from build123d import *

# Parameters (mm, degrees)
SKETCH_1_W          = 37.5
SKETCH_1_H          = 37.5
EXTRUDE_1_DEPTH     = 82
SKETCH_2_W          = 57
SKETCH_2_H          = 57
EXTRUDE_2_DEPTH     = 2
SKETCH_3_R          = 2.5
CUT_EXTRUDE_1_DEPTH = 2
SKETCH_4_R          = 4
EXTRUDE_3_DEPTH     = 23


with BuildPart() as part:
    # 草图1 → 凸台-拉伸1 (new body)
    with BuildSketch(Plane(origin=(0, 0, 0), x_dir=(1, 0, 0), z_dir=(0, 1, 0))):
        with BuildLine():
            Line((-18.75, 18.75), (-25, 18.75))
            ThreePointArc((-25, 18.75), (-27.121320344, 17.871320344), (-28, 15.75))
            Line((-28, 15.75), (-28, -15.75))
            ThreePointArc((-28, -15.75), (-27.121320344, -17.871320344), (-25, -18.75))
            Line((-25, -18.75), (-18.75, -18.75))
            Line((-18.75, -18.75), (-18.75, 18.75))
        make_face()
        Rectangle(SKETCH_1_W, SKETCH_1_H)
        with BuildLine():
            Line((25, 18.75), (18.75, 18.75))
            Line((18.75, 18.75), (18.75, -18.75))
            Line((18.75, -18.75), (25, -18.75))
            ThreePointArc((25, -18.75), (27.121320344, -17.871320344), (28, -15.75))
            Line((28, -15.75), (28, 15.75))
            ThreePointArc((28, 15.75), (27.121320344, 17.871320344), (25, 18.75))
        make_face()
        with BuildLine():
            Line((18.75, -18.75), (-18.75, -18.75))
            Line((-18.75, -18.75), (-18.75, -25))
            ThreePointArc((-18.75, -25), (-17.871320344, -27.121320344), (-15.75, -28))
            Line((-15.75, -28), (15.75, -28))
            ThreePointArc((15.75, -28), (17.871320344, -27.121320344), (18.75, -25))
            Line((18.75, -25), (18.75, -18.75))
        make_face()
        with BuildLine():
            Line((-18.75, 25), (-18.75, 18.75))
            Line((-18.75, 18.75), (18.75, 18.75))
            Line((18.75, 18.75), (18.75, 25))
            ThreePointArc((18.75, 25), (17.871320344, 27.121320344), (15.75, 28))
            Line((15.75, 28), (-15.75, 28))
            ThreePointArc((-15.75, 28), (-17.871320344, 27.121320344), (-18.75, 25))
        make_face()
    extrude(amount=EXTRUDE_1_DEPTH)

    # 草图2 → 凸台-拉伸2 (add)
    with BuildSketch(Plane(origin=(0, 82, 0), x_dir=(1, 0, 0), z_dir=(0, 1, 0))):
        Rectangle(SKETCH_2_W, SKETCH_2_H)
    extrude(amount=-EXTRUDE_2_DEPTH)

    # 草图3 → 切除-拉伸1 (cut)
    with BuildSketch(Plane(origin=(0, 82, 0), x_dir=(1, 0, 0), z_dir=(0, 1, 0))):
        with Locations((23.5, 23.5)):
            Circle(SKETCH_3_R)
        with Locations((-23.5, 23.5)):
            Circle(SKETCH_3_R)
        with Locations((-23.5, -23.5)):
            Circle(SKETCH_3_R)
        with Locations((23.5, -23.5)):
            Circle(SKETCH_3_R)
    extrude(amount=-CUT_EXTRUDE_1_DEPTH, mode=Mode.SUBTRACT)

    # 草图4 → 凸台-拉伸3 (add)
    with BuildSketch(Plane(origin=(0, 82, 0), x_dir=(1, 0, 0), z_dir=(0, 1, 0))):
        Circle(SKETCH_4_R)
    extrude(amount=EXTRUDE_3_DEPTH)


solid = part.part
Design review of the part built by this model. Coordinates are the model's own, in mm. A direction names the side the tool comes from. Round coordinates to 2 decimals unless told otherwise and drop trailing zeros. Write each loop counter-clockwise with the first axis right and the second up, starting at its lowest first coordinate (ties: lowest second). Pieces come first, ordered by that corner, then holes. Notation, with made-up numbers: (-38.75, 87.25) - (-3.75, 87.25) arc R25 ccw to (-3.75, 126.25) - close; hole circle Ø9 at (-18, 72.5). An arc over 180 degrees is marked (long way). Use a Markdown table: item, result. Add a question column.
1. We need section B-B (x = 23.5). State the section outline as (y, z) points, then the cut area to 3 significant figures.
2. Clearance check with flat-ended pins moving along their axes: pin 1 (1 mm diameter, centred on x = 1.5, y = 60.5, fed in from -Z); pin 2 (7 mm diameter, centred on y = 56, z = -22, fed in from +X); pin 3 (8 mm diameter, centred on x = 23.5, z = 23.5, fed in from -Y). State where each tip first meets the part, or that it passes through.
3. Wall thickness on probe 1 along X at (y, z) = (80.75, -23.5); probe 2 along X at (y, z) = (32, 11): over which ranges is each line inside the solid? List them lowest first.
4. We need section A-A (z = -23.5). State the section outline as (x, y) points, then the cut area to 3 significant figures.
5. Mouldability with a two-part tool opening along Z and no side actions: class faces 6 (the face through (28, 39, 0)), 7 (the face through (27.1, 39.44, 17.89)), 8 (the face through (0, 81, -28.5)), 9 (the face through (21.66, 81.01, -25.19)) as +Z half, -Z half, draft (parallel to the pull), parting line (faces both ways), or undercut.
6. We need section C-C (y = 49). State the section outline as (x, z) points, then the cut area to 3 significant figures.
7. We need section D-D (x = 0). State the section outline as (y, z) points, then the cut area to 3 significant figures.
8. For faces 1 (the face through (-0.867, 93.339, 3.905)), 2 (the face through (19, 80, 19)), 3 (the face through (-22, 39, 18.75)), 4 (the face through (22, 39, -18.75)), 5 (the face through (18.75, 39, 22)), list the 3-axis set-ups (+Z, -Z, +X, -X, +Y, -Y) from which the entire face can be reached by the end or side of a thin tool; tool diameter is ignored.
Output:
| question | item | result |
|---|---|---|
| 1 | outline | (0, -18.75) - (80, -18.75) - (80, -21) - (82, -21) - (82, 21) - (80, 21) - (80, 18.75) - (0, 18.75) - close; (80, -28.5) - (82, -28.5) - (82, -26) - (80, -26) - close; (80, 26) - (82, 26) - (82, 28.5) - (80, 28.5) - close |
| 1 | area | 3,090 mm2 |
| 2 | pin 1 | stops at z = -28 |
| 2 | pin 2 | stops at x = 26.2 |
| 2 | pin 3 | stops at y = 80 |
| 3 | probe 1 | x = -28.5 to -26, -21 to 21, 26 to 28.5 |
| 3 | probe 2 | x = -28 to 28 |
| 4 | outline | (-28.5, 80) - (-26, 80) - (-26, 82) - (-28.5, 82) - close; (-21, 80) - (-18.75, 80) - (-18.75, 0) - (18.75, 0) - (18.75, 80) - (21, 80) - (21, 82) - (-21, 82) - close; (26, 80) - (28.5, 80) - (28.5, 82) - (26, 82) - close |
| 4 | area | 3,090 mm2 |
| 5 | face 6 | draft |
| 5 | face 7 | +Z half |
| 5 | face 8 | -Z half |
| 5 | face 9 | undercut |
| 6 | outline | (-28, -15.75) arc R3 ccw to (-25, -18.75) - (-18.75, -18.75) - (-18.75, -25) arc R3 ccw to (-15.75, -28) - (15.75, -28) arc R3 ccw to (18.75, -25) - (18.75, -18.75) - (25, -18.75) arc R3 ccw to (28, -15.75) - (28, 15.75) arc R3 ccw to (25, 18.75) - (18.75, 18.75) - (18.75, 25) arc R3 ccw to (15.75, 28) - (-15.75, 28) arc R3 ccw to (-18.75, 25) - (-18.75, 18.75) - (-25, 18.75) arc R3 ccw to (-28, 15.75) - close |
| 6 | area | 2,780 mm2 |
| 7 | outline | (0, -28) - (80, -28) - (80, -28.5) - (82, -28.5) - (82, -4) - (105, -4) - (105, 4) - (82, 4) - (82, 28.5) - (80, 28.5) - (80, 28) - (0, 28) - close |
| 7 | area | 4,780 mm2 |
| 8 | face 1 | +Y |
| 8 | face 2 | -Y |
| 8 | face 3 | +Z, -X, -Y |
| 8 | face 4 | -Z, +X, -Y |
| 8 | face 5 | +Z, +X, -Y |
